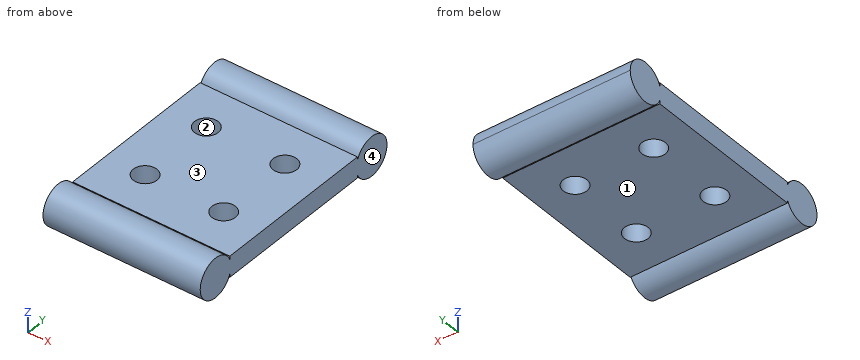
```python
from build123d import *

# Parameters (mm, degrees)
F0_W     = 60
F0_H     = 62.5
F1_DEPTH = 8
F3_D     = 9
F3_DEPTH = 15
F3_TIP   = 2.7038727856
F5_DEPTH = 60


with BuildPart() as f1:
    # F0 (on Top) → F1 (new body)
    with BuildSketch(Plane.XY):
        with Locations((30, -31.25)):
            Rectangle(F0_W, F0_H)
    extrude(amount=F1_DEPTH)

    # F3
    with Locations(Plane.XY.offset(8)):
        with Locations((15, -16.25), (45, -16.25), (45, -46.25), (15, -46.25)):
            Hole(F3_D / 2, depth=F3_DEPTH)
            with Locations((0, 0, -(F3_DEPTH + F3_TIP / 2))):  # 118° drill point
                Cone(0, F3_D / 2, F3_TIP, mode=Mode.SUBTRACT)

    # F4 (on face) → F5 (join)
    with BuildSketch(Plane.YZ.offset(60)):
        with BuildLine():
            ThreePointArc((-62.5, 1.3074175964), (-62.1260593981, 2.6306936062), (-62, 4))
            ThreePointArc((-62, 4), (-62.1260593981, 5.3693063938), (-62.5, 6.6925824036))
            Line((-62.5, 6.6925824036), (-62.5, 1.3074175964))
        make_face()
        with BuildLine():
            Line((-62.5, 1.3074175964), (-62.5, 6.6925824036))
            ThreePointArc((-62.5, 6.6925824036), (-77, 4), (-62.5, 1.3074175964))
        make_face()
        with BuildLine():
            ThreePointArc((14.5, 4), (8.3693063938, 11.3739406019), (0, 6.6925824036))
            Line((0, 6.6925824036), (0, 1.3074175964))
            ThreePointArc((0, 1.3074175964), (8.3693063938, -3.3739406019), (14.5, 4))
        make_face()
    extrude(amount=-F5_DEPTH)


solid = f1.part
```
Geometry check sheet. Reference: the model listing, model coordinates, mm. Face numbers are marked on the shaded views. A direction names the side the tool comes from. Round coordinates to 2 decimals unless told otherwise and drop trailing zeros. Order: outer loops, then holes, each group sorted by start corner. A loop starts at its lowest first (then second) coordinate and runs counter-clockwise, first axis right, second up. Notation, with made-up numbers: M 46.5,-13.75 L 62.5,-13.75 A13 cw 62.5,-4.75 Z; hole C -24,73 d7. An arc over 180 degrees is marked long. Write item = value, one per line.
Q1. Scan lines: line 1 (Y direction, x = 15, z = 4.5); line 2 (Y direction, x = 15, z = 5.25); line 3 (X direction, y = -43, z = 7). Record each from-to range of solid material in increasing order.
Answer block:
line_1 = -76.98 to -50.75, -41.75 to -20.75, -11.75 to 14.48
line_2 = -76.9 to -50.75, -41.75 to -20.75, -11.75 to 14.4
line_3 = 0 to 11.89, 18.11 to 41.89, 48.11 to 60
Q2. Section check B-B (x = 45). Enter the section's corners in (y, z).
Answer block:
outline = M -62.5,0 L -50.75,0 L -50.75,8 L -62.5,8 L -62.5,6.69 A7.5 ccw long -62.5,1.31 Z; M -41.75,0 L -20.75,0 L -20.75,8 L -41.75,8 Z; M -11.75,0 L 0,0 L 0,1.31 A7.5 ccw long 0,6.69 L 0,8 L -11.75,8 Z
Q3. Release check for a two-part mould opening along Y. For the marked faces 3 and 4 record: released by +Y, released by -Y, zero draft, split by the parting line, or undercut.
Answer block:
face_3 = undercut
face_4 = zero draft
Q4. Section check A-A (y = -46.25). Enter the section's corners in (x, z).
Answer block:
outline = M 0,0 L 10.5,0 L 10.5,8 L 0,8 Z; M 19.5,0 L 40.5,0 L 40.5,8 L 19.5,8 Z; M 49.5,0 L 60,0 L 60,8 L 49.5,8 Z
Q5. Set-up check for the marked faces 1 and 2: record each of +Z, -Z, +X, -X, +Y, -Y from which the full face is reachable in a straight line by a thin tool's end or side.
Answer block:
face_1 = -Z, +X, -X
face_2 = +Z, -Z
Q6. Section check D-D (y = -58.5). Enter the section's corners in (x, z).
Answer block:
outline = M 0,0 L 60,0 L 60,8 L 0,8 Z
Q7. Depth check by flat-ended pin: pin 1 Ø10 at (x, y) = (22, -33.5) entering from -Z; pin 2 Ø7 at (x, y) = (15, -46.25) entering from +Z; pin 3 Ø6 at (x, y) = (39.5, -9.5) entering from +Z; pin 4 Ø1 at (x, z) = (18.5, 7) entering from +Y. Enter the tip coordinate at first touch or a pass-through.
Answer block:
pin_1 = 0
pin_2 = through
pin_3 = 8
pin_4 = 14.07
Q8. Section check C-C (x = 5). Enter the section's corners in (y, z), plus the area to 3 significant figures.
Answer block:
outline = M -62.5,0 L 0,0 L 0,1.31 A7.5 ccw long 0,6.69 L 0,8 L -62.5,8 L -62.5,6.69 A7.5 ccw long -62.5,1.31 Z
area = 850 mm^2
